from build123d import *

# Parameters (mm, degrees)
SKETCH1_W                                       = 63.5
SKETCH1_H                                       = 63.5
BOSS_EXTRUDE1_DEPTH                             = 3.175
CUT_EXTRUDE1_REACH                              = 47.013
SKETCH2_R                                       = 14.3129
CSK_FOR_M5_FLAT_HEAD_MACHINE_SCREW1_D           = 5.8
CSK_FOR_M5_FLAT_HEAD_MACHINE_SCREW1_DEPTH       = 6.35
CSK_FOR_M5_FLAT_HEAD_MACHINE_SCREW1_CSINK_D     = 10.4
CSK_FOR_M5_FLAT_HEAD_MACHINE_SCREW1_CSINK_ANGLE = 90
CSK_FOR_M5_FLAT_HEAD_MACHINE_SCREW1_TIP         = 1.742495795
FILLET1_R                                       = 3.175
CUT_EXTRUDE2_REACH                              = 47.013
SKETCH5_R                                       = 2.6162


with BuildPart() as part:
    # Sketch1 → Boss-Extrude1 (new body)
    with BuildSketch(Plane(origin=(0, 0, 0), x_dir=(1, 0, 0), z_dir=(0, 1, 0))):
        Rectangle(SKETCH1_W, SKETCH1_H)
    extrude(amount=BOSS_EXTRUDE1_DEPTH)

    # Sketch2 → Cut-Extrude1 (cut, up to next)
    with BuildSketch(Plane(origin=(0, 3.175, 0), x_dir=(1, 0, 0), z_dir=(0, 1, 0)), mode=Mode.PRIVATE) as cut_extrude1_sk1:
        with Locations(Location((0, 0, 0), (0, 0, 270))):
            Circle(SKETCH2_R)
    cut_extrude1_tool1 = extrude(cut_extrude1_sk1.sketch, amount=-CUT_EXTRUDE1_REACH, mode=Mode.PRIVATE) & part.part
    add(cut_extrude1_tool1.solids().sort_by_distance((0, 3.175, 0))[0], mode=Mode.SUBTRACT)

    # CSK for M5 Flat Head Machine Screw1
    with Locations(Plane(origin=(-14.368409794, 0, 14.368409794), x_dir=(0, 0, -1), z_dir=(0, -1, 0))):
        with Locations((0, 0), (0, 28.736819588), (28.736819588, 28.736819588), (28.736819588, 0)):
            CounterSinkHole(CSK_FOR_M5_FLAT_HEAD_MACHINE_SCREW1_D / 2, CSK_FOR_M5_FLAT_HEAD_MACHINE_SCREW1_CSINK_D / 2, depth=CSK_FOR_M5_FLAT_HEAD_MACHINE_SCREW1_DEPTH, counter_sink_angle=CSK_FOR_M5_FLAT_HEAD_MACHINE_SCREW1_CSINK_ANGLE)
            with Locations((0, 0, -(CSK_FOR_M5_FLAT_HEAD_MACHINE_SCREW1_DEPTH + CSK_FOR_M5_FLAT_HEAD_MACHINE_SCREW1_TIP / 2))):  # 118° drill point
                Cone(0, CSK_FOR_M5_FLAT_HEAD_MACHINE_SCREW1_D / 2, CSK_FOR_M5_FLAT_HEAD_MACHINE_SCREW1_TIP, mode=Mode.SUBTRACT)

    # Fillet1
    fillet1_edges = [part.edges().sort_by_distance(p)[0] for p in [
        (-31.75, 1.5875, -31.75),
        (31.75, 1.5875, -31.75),
        (31.75, 1.5875, 31.75),
        (-31.75, 1.5875, 31.75),
    ]]
    fillet(fillet1_edges, radius=FILLET1_R)

    # Sketch5 → Cut-Extrude2 (cut, up to next)
    with BuildSketch(Plane(origin=(0, 0, 0), x_dir=(-1, 0, 0), z_dir=(0, -1, 0)), mode=Mode.PRIVATE) as cut_extrude2_sk1:
        with Locations(Location((-26.042742751, -26.042742751, 0), (0, 0, 90))):
            Circle(SKETCH5_R)
    cut_extrude2_tool1 = extrude(cut_extrude2_sk1.sketch, amount=-CUT_EXTRUDE2_REACH, mode=Mode.PRIVATE) & part.part
    # Sketch5 → Cut-Extrude2 (cut, up to next)
    with BuildSketch(Plane(origin=(0, 0, 0), x_dir=(-1, 0, 0), z_dir=(0, -1, 0)), mode=Mode.PRIVATE) as cut_extrude2_sk2:
        with Locations(Location((-26.042742751, 26.042742751, 0), (0, 0, 90))):
            Circle(SKETCH5_R)
    cut_extrude2_tool2 = extrude(cut_extrude2_sk2.sketch, amount=-CUT_EXTRUDE2_REACH, mode=Mode.PRIVATE) & part.part
    # Sketch5 → Cut-Extrude2 (cut, up to next)
    with BuildSketch(Plane(origin=(0, 0, 0), x_dir=(-1, 0, 0), z_dir=(0, -1, 0)), mode=Mode.PRIVATE) as cut_extrude2_sk3:
        with Locations(Location((26.042742751, 26.042742751, 0), (0, 0, 90))):
            Circle(SKETCH5_R)
    cut_extrude2_tool3 = extrude(cut_extrude2_sk3.sketch, amount=-CUT_EXTRUDE2_REACH, mode=Mode.PRIVATE) & part.part
    # Sketch5 → Cut-Extrude2 (cut, up to next)
    with BuildSketch(Plane(origin=(0, 0, 0), x_dir=(-1, 0, 0), z_dir=(0, -1, 0)), mode=Mode.PRIVATE) as cut_extrude2_sk4:
        with Locations(Location((26.042742751, -26.042742751, 0), (0, 0, 90))):
            Circle(SKETCH5_R)
    cut_extrude2_tool4 = extrude(cut_extrude2_sk4.sketch, amount=-CUT_EXTRUDE2_REACH, mode=Mode.PRIVATE) & part.part
    add(cut_extrude2_tool1.solids().sort_by_distance((26.042743, 0, 26.042743))[0], mode=Mode.SUBTRACT)
    add(cut_extrude2_tool2.solids().sort_by_distance((26.042743, 0, -26.042743))[0], mode=Mode.SUBTRACT)
    add(cut_extrude2_tool3.solids().sort_by_distance((-26.042743, 0, -26.042743))[0], mode=Mode.SUBTRACT)
    add(cut_extrude2_tool4.solids().sort_by_distance((-26.042743, 0, 26.042743))[0], mode=Mode.SUBTRACT)


solid = part.part
Check sheet for the modelled part. Datum: model origin and axes. Units: mm. Round coordinates to 2 decimals unless told otherwise and drop trailing zeros. Loops run counter-clockwise (first coordinate to the right, second up) from the corner with the lowest first, then second, coordinate; pieces in that order, holes last. Notation, with made-up numbers: (29, 13) -> (73, 13) arc R23 ccw to (73, 37) -> close; hole circle Ø2 at (82.25, 5.25). An arc over 180 degrees is marked (long way). Put each result on its own line as item: value. Start each with the question number.
1. Section check B-B (z = 0). Enter the section's corners in (x, y) (3 decimals).
2. Section check C-C (y = 0.6). Give the number of separate pieces and of enclosed holes in the cut face, plus the area to 3 significant figures.
3. Scan lines: probe 1 along X at (y, z) = (2.2, -26); probe 2 along Z at (x, y) = (-13, 2.45); probe 3 along X at (y, z) = (0.85, 24). Record each from-to range of solid material in increasing order.
4. Section check A-A (x = 0). Enter the section's corners in (y, z) (3 decimals), plus the area to 3 significant figures.
5. Section check D-D (z = 26.5). Enter the section's corners in (x, y) (3 decimals), plus the area to 3 significant figures.
6. Draft check along Z on faces 1 (the face through (0, 2, -31.75)), 2 (the face through (15.239, 2.744, -11.602)), 3 (the face through (-30.84, 1.61, 30.8)), 4 (the face through (-31.75, 2, 0)). Enter one of: +Z half, -Z half, draft (parallel to the pull), parting line (faces both ways), or undercut.
7. Gauge pin test, flat ends, axial feed: pin 1 (7 mm diameter, centred on x = -26.04, z = 26.04, fed in from -Y); pin 2 (4.5 mm diameter, centred on x = 26.04, z = -26.04, fed in from -Y); pin 3 (9.5 mm diameter, centred on x = 14.37, z = -14.37, fed in from -Y). Record the tip position at first contact, or that the pin passes through.
Findings:
1. outline: (-31.75, 0) -> (-14.313, 0) -> (-14.313, 3.175) -> (-31.75, 3.175) -> close; (14.313, 0) -> (31.75, 0) -> (31.75, 3.175) -> (14.313, 3.175) -> close
2. separate pieces: 1
2. enclosed holes: 9
2. area: 3,030 mm^2
3. probe 1: x = -31.75 to -28.66, -23.43 to 23.43, 28.66 to 31.75
3. probe 2: z = -31.75 to -16.93, -11.81 to -5.99, 5.99 to 11.81, 16.93 to 31.75
3. probe 3: x = -31.75 to -27.68, -24.41 to 24.41, 27.68 to 31.75
4. outline: (0, -31.75) -> (3.175, -31.75) -> (3.175, -14.313) -> (0, -14.313) -> close; (0, 14.313) -> (3.175, 14.313) -> (3.175, 31.75) -> (0, 31.75) -> close
4. area: 111 mm^2
5. outline: (-31.75, 0) -> (-28.619, 0) -> (-28.619, 3.175) -> (-31.75, 3.175) -> close; (-23.467, 0) -> (23.467, 0) -> (23.467, 3.175) -> (-23.467, 3.175) -> close; (28.619, 0) -> (31.75, 0) -> (31.75, 3.175) -> (28.619, 3.175) -> close
5. area: 169 mm^2
6. face 1: -Z half
6. face 2: undercut
6. face 3: +Z half
6. face 4: draft
7. pin 1: stops at y = 0
7. pin 2: passes through
7. pin 3: stops at y = 0.45
